Work out the finished part from the listing and answer in its coordinate system (mm). A direction names the side the tool comes from. Round coordinates to 2 decimals unless told otherwise and drop trailing zeros. Loops run counter-clockwise (first coordinate to the right, second up) from the corner with the lowest first, then second, coordinate; pieces in that order, holes last.
Autodesk Fusion 360 part; units mm, degrees
sketch "Skizze2" plane through (0, 0, 0) normal (0, 0, 1) x (1, 0, 0)
  circle A0 centre (0, 0) radius 16
  dimension "d2" = 32
extrude "Extrusion1" add sketch "Skizze2" along normal blind 12.5
sketch "Skizze3" plane through (0, 0, 12.5) normal (0, 0, 1) x (-1, 0, 0)
  circle A0 centre (0, 0) radius 16
  circle A1 centre (0, 0) radius 15
  dimension "d5" = 30
extrude "Extrusion2" add sketch "Skizze3" along normal blind 7 contours A1
sketch "Skizze4" plane through (0, 0, 19.5) normal (0, 0, 1) x (-1, 0, 0)
  circle A0 centre (0, 0) radius 15
  circle A1 centre (0, 0) radius 11.75
  dimension "d8" = 23.5
extrude "Extrusion3" cut sketch "Skizze4" against normal blind 10 contours A1
sketch "Skizze5" plane through (0, 0, 9.5) normal (0, 0, 1) x (-1, 0, 0)
  circle A0 centre (0, 0) radius 11.75
  circle A1 centre (0, 0) radius 1.15
  dimension "d11" = 2.3
extrude "Extrusion4" cut sketch "Skizze5" against normal blind 300 contours A1
sketch "Skizze6" plane through (0, 0, 0) normal (0, 0, -1) x (1, 0, 0)
  circle A0 centre (0, 0) radius 1.15
  circle A1 centre (0, 0) radius 16
  circle A2 centre (0, 0) radius 12.5
  dimension "d14" = 25
extrude "Extrusion5" cut sketch "Skizze6" against normal blind 5 contours A2
sketch "Skizze7" plane through (0, 0, 5) normal (0, 0, -1) x (1, 0, 0)
  circle A0 centre (0, 0) radius 1.15
  circle A1 centre (0, 0) radius 12.5
  circle A2 centre (0, -4.5) radius 1
  dimension "d17" = 2
extrude "Extrusion6" cut sketch "Skizze7" against normal blind 300 contours A2
sketch "Skizze8" plane through (0, 0, 5) normal (0, 0, -1) x (1, 0, 0)
  circle A0 centre (0, -4.5) radius 1
  circle A1 centre (0, 0) radius 1.15
  circle A2 centre (0, 0) radius 12.5
  circle A3 centre (4.5, 0) radius 1
  dimension "d20" = 2
extrude "Extrusion7" cut sketch "Skizze8" against normal blind 300 contours A3
sketch "Skizze9" plane through (0, 0, 5) normal (0, 0, -1) x (1, 0, 0)
  circle A0 centre (4.5, 0) radius 1
  circle A1 centre (0, -4.5) radius 1
  circle A2 centre (0, 0) radius 1.15
  circle A3 centre (0, 0) radius 12.5
  circle A4 centre (0, 4.5) radius 1
  dimension "d23" = 2
extrude "Extrusion8" cut sketch "Skizze9" against normal blind 300 contours A4
sketch "Skizze10" plane through (0, 0, 5) normal (0, 0, -1) x (1, 0, 0)
  circle A0 centre (0, 4.5) radius 1
  circle A1 centre (4.5, 0) radius 1
  circle A2 centre (0, -4.5) radius 1
  circle A3 centre (0, 0) radius 1.15
  circle A4 centre (0, 0) radius 12.5
  circle A5 centre (-4.5, 0) radius 1
  dimension "d26" = 2
extrude "Extrusion9" cut sketch "Skizze10" against normal blind 300 contours A5
1. Find section D-D (y = -4.5). Write down the section's boundary in (x, z).
Answer key:
outline: (-15.35, 0) - (-11.66, 0) - (-11.66, 5) - (-1, 5) - (-1, 9.5) - (-10.85, 9.5) - (-10.85, 19.5) - (-14.31, 19.5) - (-14.31, 12.5) - (-15.35, 12.5) - close; (1, 5) - (11.66, 5) - (11.66, 0) - (15.35, 0) - (15.35, 12.5) - (14.31, 12.5) - (14.31, 19.5) - (10.85, 19.5) - (10.85, 9.5) - (1, 9.5) - close
2. Which of the six approach directions +Z, -Z, +X, -X, +Y, -Y give full straight-line access (tool end or side, diameter ignored) to faces 1 (the face through (9, 8, 19.5)), 2 (the face through (0, 2, 9.5)), 3 (the face through (11.923, -3.755, 2.465))?
Answer key:
face 1: +Z, +X, -X, +Y, -Y
face 2: +Z
face 3: -Z
3. Determine the mould class of faces 4 (the face through (-0.13, -5.49, 7.22)), 5 (the face through (-10, -8, 0)), 6 (the face through (0, 3, 5)), 7 (the face through (14.985, 0.66, 15.951)) for opening direction Y: +Y half, -Y half, draft (parallel to the pull), parting line (faces both ways), or undercut.
Answer key:
face 4: undercut
face 5: draft
face 6: undercut
face 7: parting line
4. Consider probe 1 along Y at (x, z) = (0, 6.55); probe 2 along Y at (x, z) = (0, 3.1); probe 3 along Y at (x, z) = (0, 17). Determine where each line is inside the solid, lowest interval first.
Answer key:
probe 1: y = -16 to -5.5, -3.5 to -1.15, 1.15 to 3.5, 5.5 to 16
probe 2: y = -16 to -12.5, 12.5 to 16
probe 3: y = -15 to -11.75, 11.75 to 15
5. Find section C-C (z = 7). Write down the section's boundary in (x, y).
Answer key:
outline: circle Ø32 at (0, 0); hole circle Ø2 at (-4.5, 0); hole circle Ø2.3 at (0, 0); hole circle Ø2 at (0, -4.5); hole circle Ø2 at (0, 4.5); hole circle Ø2 at (4.5, 0)
6. Given pin 1 (2.5 mm diameter, centred on x = 0, y = 0, fed in from +Z); pin 2 (10 mm diameter, centred on y = 6, z = 5, fed in from +X); pin 3 (7.5 mm diameter, centred on x = -1.5, y = 1, fed in from -Z), each flat-ended and moving along its own axis, determine where each tip first touches the part or whether it passes through.
Answer key:
pin 1: stops at z = 9.5
pin 2: stops at x = 15.97
pin 3: stops at z = 5
7. Find section A-A (x = 0). Write down the section's boundary in (y, z).
Answer key:
outline: (-16, 0) - (-12.5, 0) - (-12.5, 5) - (-5.5, 5) - (-5.5, 9.5) - (-11.75, 9.5) - (-11.75, 19.5) - (-15, 19.5) - (-15, 12.5) - (-16, 12.5) - close; (-3.5, 5) - (-1.15, 5) - (-1.15, 9.5) - (-3.5, 9.5) - close; (1.15, 5) - (3.5, 5) - (3.5, 9.5) - (1.15, 9.5) - close; (5.5, 5) - (12.5, 5) - (12.5, 0) - (16, 0) - (16, 12.5) - (15, 12.5) - (15, 19.5) - (11.75, 19.5) - (11.75, 9.5) - (5.5, 9.5) - close
